Geometry: final body of the model. Coordinates: model frame, mm. A direction names the side the tool comes from. Coordinates: 2 decimals unless noted, no trailing zeros. Order: outer loops, then holes, each group sorted by start corner. A loop starts at its lowest first (then second) coordinate and runs counter-clockwise, first axis right, second up. Notation, with made-up numbers: (17, -27) -> (31, -27) arc R26 cw to (31, -4) -> close; hole circle Ø5 at (35, 82.5). An arc over 180 degrees is marked (long way). Answer in a Markdown table with one row per item. Add a question column.
1) Section query C-C on x = -2.45. Return the cut outline in (y, z), then the cut area to 3 significant figures.
2) Section query D-D on y = 1.25. Return the cut outline in (x, z), then the cut area to 3 significant figures.
3) Ray query, line 1 (Z direction, x = 0, y = 6.5); line 2 (Z direction, x = 0, y = 4.7). Return the intervals inside material, ascending. Write a range as from..to.
4) Set-up query: faces 1 (the face through (0, 6, 2)), 2 (the face through (0, 0, 0)). Return all of +Z, -Z, +X, -X, +Y, -Y with unobstructed straight access to the full face (end or side cutting, diameter ignored); none if empty.
5) Contact query for flat-ended pins moving along their axis: P1, Ø3, axis at y = 7, z = 1.5, coming from the -X side; P2, Ø1, axis at x = 0.5, z = -1, coming from the -Y side. Output: stop coordinate, or through.
6) Pull-direction query (X, two-part tool) for faces 3 (the face through (-1, 8, -1)), 4 (the face through (-0.875, 4.958, 0.558)), 5 (the face through (-1.717, 6.986, -0.541)); classes: +X half, -X half, draft (parallel to the pull), parting line (faces both ways), or undercut.
7) Section query B-B on z = -1.45. Return the cut outline in (x, y).
8) Section query A-A on y = 3.25. Return the cut outline in (x, z).
Autodesk Fusion 360 part; units mm, degrees
sketch "Sketch1" plane through (0, 0, 0) normal (0, 1, 0) x (1, 0, 0)
  circle A0 centre (0, 0) radius 3
extrude "Extrude1" add sketch "Sketch1" along normal blind 6
sketch "Sketch2" plane through (0, 6, 0) normal (0, 1, 0) x (-1, 0, 0)
  circle A0 centre (0, 0) radius 3
  circle A1 centre (0, 0) radius 1.8
extrude "Extrude2" add sketch "Sketch2" along normal blind 2 contours A1
hole "Hole1" at (0, 8, 0) direction (0, -1, 0) diameter 2.076 depth 6 tip angle 118
Result:
| question | item | result |
|---|---|---|
| 1 | outline | (0, -1.73) -> (6, -1.73) -> (6, 1.73) -> (0, 1.73) -> close |
| 1 | area | 20.8 mm2 |
| 2 | outline | circle Ø6 at (0, 0) |
| 2 | area | 28.3 mm2 |
| 3 | line 1 | -1.8..-1.04, 1.04..1.8 |
| 3 | line 2 | -3..-1.04, 1.04..3 |
| 4 | face 1 | +Y |
| 4 | face 2 | +Z, -Z, +X, -X, -Y |
| 5 | P1 | x = -2.98 |
| 5 | P2 | y = 0 |
| 6 | face 3 | draft |
| 6 | face 4 | undercut |
| 6 | face 5 | parting line |
| 7 | outline | (-2.63, 0) -> (2.63, 0) -> (2.63, 6) -> (1.07, 6) -> (1.07, 8) -> (-1.07, 8) -> (-1.07, 6) -> (-2.63, 6) -> close |
| 8 | outline | circle Ø6 at (0, 0); hole circle Ø2.08 at (0, 0) |
